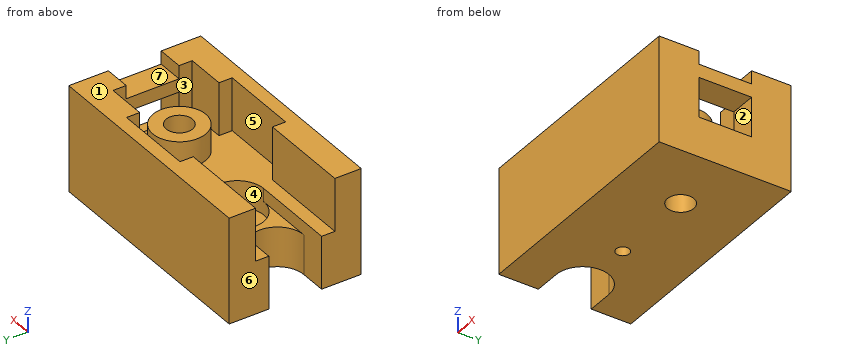
```python
from build123d import *

# Parameters (mm, degrees)
SKETCH1_W           = 180
SKETCH1_H           = 100
BOSS_EXTRUDE1_DEPTH = 80
CUT_EXTRUDE1_DEPTH  = 80
SKETCH3_R           = 5
CUT_EXTRUDE2_DEPTH  = 20
SKETCH4_R           = 10
CUT_EXTRUDE3_DEPTH  = 60
SKETCH5_R           = 20
CUT_EXTRUDE4_DEPTH  = 60
SKETCH6_R           = 20
CUT_EXTRUDE5_DEPTH  = 50
CUT_EXTRUDE6_DEPTH  = 50
SKETCH8_W           = 10
SKETCH8_H           = 40
CUT_EXTRUDE7_DEPTH  = 207
CUT_EXTRUDE8_DEPTH  = 10
CUT_EXTRUDE9_DEPTH  = 10
SKETCH11_W          = 20
SKETCH11_H          = 40
CUT_EXTRUDE10_DEPTH = 30
SKETCH12_R          = 20
SKETCH12_R_2        = 10
BOSS_EXTRUDE3_DEPTH = 30
SKETCH13_R          = 20
CUT_EXTRUDE11_DEPTH = 30
SKETCH14_W          = 20
SKETCH14_H          = 40
CUT_EXTRUDE12_DEPTH = 10
SKETCH15_W          = 10
SKETCH15_H          = 40
BOSS_EXTRUDE5_DEPTH = 20


with BuildPart() as part:
    # Sketch1 → Boss-Extrude1 (new body)
    with BuildSketch(Plane.XY):
        with Locations((90, 50)):
            Rectangle(SKETCH1_W, SKETCH1_H)
    extrude(amount=BOSS_EXTRUDE1_DEPTH)

    # Sketch2 → Cut-Extrude1 (cut)
    with BuildSketch(Plane.XY.offset(80)):
        with BuildLine():
            Line((0, 70), (20, 70))
            ThreePointArc((20, 70), (40, 50), (20, 30))
            Line((20, 30), (0, 30))
            Line((0, 30), (0, 70))
        make_face()
    extrude(amount=-CUT_EXTRUDE1_DEPTH, mode=Mode.SUBTRACT)

    # Sketch3 → Cut-Extrude2 (cut)
    with BuildSketch(Plane(origin=(0, 0, 0), x_dir=(-1, 0, 0), z_dir=(0, 0, -1))):
        with Locations((-65, 50)):
            Circle(SKETCH3_R)
    extrude(amount=-CUT_EXTRUDE2_DEPTH, mode=Mode.SUBTRACT)

    # Sketch4 → Cut-Extrude3 (cut)
    with BuildSketch(Plane(origin=(0, 0, 0), x_dir=(-1, 0, 0), z_dir=(0, 0, -1))):
        with Locations((-130, 50)):
            Circle(SKETCH4_R)
    extrude(amount=-CUT_EXTRUDE3_DEPTH, mode=Mode.SUBTRACT)

    # Sketch5 → Cut-Extrude4 (cut)
    with BuildSketch(Plane.XY.offset(80)):
        with Locations((65, 50)):
            Circle(SKETCH5_R)
    extrude(amount=-CUT_EXTRUDE4_DEPTH, mode=Mode.SUBTRACT)

    # Sketch6 → Cut-Extrude5 (cut)
    with BuildSketch(Plane.XY.offset(80)):
        with Locations((130, 50)):
            Circle(SKETCH6_R)
    extrude(amount=-CUT_EXTRUDE5_DEPTH, mode=Mode.SUBTRACT)

    # Sketch7 → Cut-Extrude6 (cut)
    with BuildSketch(Plane.XY.offset(80)):
        with BuildLine():
            Line((20, 70), (65, 70))
            ThreePointArc((65, 70), (45, 50), (65, 30))
            Line((65, 30), (20, 30))
            ThreePointArc((20, 30), (40, 50), (20, 70))
        make_face()
    extrude(amount=-CUT_EXTRUDE6_DEPTH, mode=Mode.SUBTRACT)

    # Sketch8 → Cut-Extrude7 (cut)
    with BuildSketch(Plane(origin=(180, 0, 0), x_dir=(0, 0, -1), z_dir=(1, 0, 0))):
        with Locations((-75, 50)):
            Rectangle(SKETCH8_W, SKETCH8_H)
    extrude(amount=-CUT_EXTRUDE7_DEPTH, mode=Mode.SUBTRACT)

    # Sketch9 → Cut-Extrude8 (cut)
    with BuildSketch(Plane.XY.offset(80)):
        Polygon((0, 70), (160, 70), (160, 80), (130, 80), (130, 90), (70, 90), (70, 80), (0, 80), align=None)
    extrude(amount=-CUT_EXTRUDE8_DEPTH, mode=Mode.SUBTRACT)

    # Sketch10 → Cut-Extrude9 (cut)
    with BuildSketch(Plane.XY.offset(80)):
        Polygon((160, 20), (160, 30), (0, 30), (0, 20), (70, 20), (70, 10), (130, 10), (130, 20), align=None)
    extrude(amount=-CUT_EXTRUDE9_DEPTH, mode=Mode.SUBTRACT)

    # Sketch11 → Cut-Extrude10 (cut)
    with BuildSketch(Plane.XY.offset(70)):
        with Locations((170, 50)):
            Rectangle(SKETCH11_W, SKETCH11_H)
    extrude(amount=-CUT_EXTRUDE10_DEPTH, mode=Mode.SUBTRACT)

    # Sketch12 → Boss-Extrude3 (add)
    with BuildSketch(Plane.XY.offset(30)):
        with Locations((130, 50)):
            Circle(SKETCH12_R)
        with Locations(Location((130, 50, 0), (0, 0, 180))):
            Circle(SKETCH12_R_2, mode=Mode.SUBTRACT)
    extrude(amount=BOSS_EXTRUDE3_DEPTH)

    # Sketch13 → Cut-Extrude11 (cut)
    with BuildSketch(Plane.XY.offset(70)):
        with BuildLine():
            Line((130, 20), (160, 20))
            Line((160, 20), (160, 30))
            Line((160, 30), (160, 70))
            Line((160, 70), (160, 80))
            Line((160, 80), (130, 80))
            Line((130, 80), (130, 90))
            Line((130, 90), (70, 90))
            Line((70, 90), (70, 80))
            Line((70, 80), (0, 80))
            Line((0, 80), (0, 70))
            Line((0, 70), (65, 70))
            ThreePointArc((65, 70), (85, 50), (65, 30))
            Line((65, 30), (0, 30))
            Line((0, 30), (0, 20))
            Line((0, 20), (70, 20))
            Line((70, 20), (70, 10))
            Line((70, 10), (130, 10))
            Line((130, 10), (130, 20))
        make_face()
        with Locations((130, 50)):
            Circle(SKETCH13_R, mode=Mode.SUBTRACT)
    extrude(amount=-CUT_EXTRUDE11_DEPTH, mode=Mode.SUBTRACT)

    # Sketch14 → Cut-Extrude12 (cut)
    with BuildSketch(Plane.XY.offset(40)):
        with Locations((170, 50)):
            Rectangle(SKETCH14_W, SKETCH14_H)
    extrude(amount=-CUT_EXTRUDE12_DEPTH, mode=Mode.SUBTRACT)

    # Sketch15 → Boss-Extrude5 (add)
    with BuildSketch(Plane.ZY.offset(-160)):
        with Locations((65, 50)):
            Rectangle(SKETCH15_W, SKETCH15_H)
    extrude(amount=-BOSS_EXTRUDE5_DEPTH)


solid = part.part
```
The listing builds one solid part. Answer for the finished solid, in the listing's coordinates (mm). Face numbers are marked on the shaded views. A direction names the side the tool comes from. Give positions to 0.01 mm unless a question says otherwise; leave off trailing zeros. Write each loop counter-clockwise with the first axis right and the second up, starting at its lowest first coordinate (ties: lowest second). Pieces come first, ordered by that corner, then holes. Notation, with made-up numbers: (-29, -13) -> (-16, -13) arc R32 ccw to (-16, 14) -> close; hole circle Ø6 at (53, -16.75). An arc over 180 degrees is marked (long way). Use one line per item in the form item = value.
1) A tool of negligible diameter and unlimited length cuts with its end or side. For the marked faces 1, 2, 3 and 4, from which of +Z, -Z, +X, -X, +Y, -Y can it reach the whole face along a straight path? Write none if from no direction.
Result:
face_1 = +Z, +X, -X, +Y, -Y
face_2 = +X
face_3 = +Z, -X
face_4 = +Z
2) Each of these flat-tipped pins is pushed along its axis until it touches: P1, Ø3, axis at y = 59.5, z = 35.5, coming from the +X side; P2, Ø16, axis at x = 168.5, y = 42, coming from the +Z side; P3, Ø4, axis at x = 21.5, z = 22, coming from the -Y side; P4, Ø8, axis at y = 62.5, z = 69, coming from the -X side. Where does it stop, or does it pass through?
Result:
P1 = 160
P2 = 70
P3 = 0
P4 = 160
3) Straight lines are drawn through the part: probe 1 along X at (y, z) = (50, 23); probe 2 along Y at (x, z) = (65, 10); probe 3 along Y at (x, z) = (16, 47). For each, find the intervals that lie inside material, in ascending order.
Result:
probe_1 = 40 to 45, 85 to 120, 140 to 180
probe_2 = 0 to 45, 55 to 100
probe_3 = 0 to 20, 80 to 100
4) Section C-C on z = 17 is taken. Write down the section's boundary in (x, y), plus the area to 3 significant figures.
Result:
outline = (0, 0) -> (180, 0) -> (180, 100) -> (0, 100) -> (0, 70) -> (20, 70) arc R20 cw to (20, 30) -> (0, 30) -> close; hole circle Ø10 at (65, 50); hole circle Ø20 at (130, 50)
area = 16,200 mm²
5) Section B-B on y = 50 is taken. Write down the section's boundary in (x, z), plus the area to 3 significant figures.
Result:
outline = (40, 0) -> (60, 0) -> (60, 20) -> (45, 20) -> (45, 30) -> (40, 30) -> close; (70, 0) -> (120, 0) -> (120, 60) -> (110, 60) -> (110, 40) -> (85, 40) -> (85, 20) -> (70, 20) -> close; (140, 0) -> (180, 0) -> (180, 30) -> (160, 30) -> (160, 40) -> (150, 40) -> (150, 60) -> (140, 60) -> close; (160, 60) -> (180, 60) -> (180, 70) -> (160, 70) -> close
area = 4,150 mm²
6) Section D-D on x = 153 is taken. Write down the section's boundary in (y, z), plus the area to 3 significant figures.
Result:
outline = (0, 0) -> (100, 0) -> (100, 80) -> (80, 80) -> (80, 40) -> (20, 40) -> (20, 80) -> (0, 80) -> close
area = 5,600 mm²
7) For a pull along X with two mould halves and no side action, classify the marked faces 5, 6 and 7 as +X half, -X half, draft (parallel to the pull), parting line (faces both ways), or undercut.
Result:
face_5 = undercut
face_6 = -X half
face_7 = draft
8) Section A-A on z = 56 is taken. Write down the section's boundary in (x, y).
Result:
outline = (0, 0) -> (180, 0) -> (180, 30) -> (160, 30) -> (160, 20) -> (130, 20) -> (130, 10) -> (70, 10) -> (70, 20) -> (0, 20) -> close; (0, 80) -> (70, 80) -> (70, 90) -> (130, 90) -> (130, 80) -> (160, 80) -> (160, 70) -> (180, 70) -> (180, 100) -> (0, 100) -> close; circle Ø40 at (130, 50); hole circle Ø20 at (130, 50)
